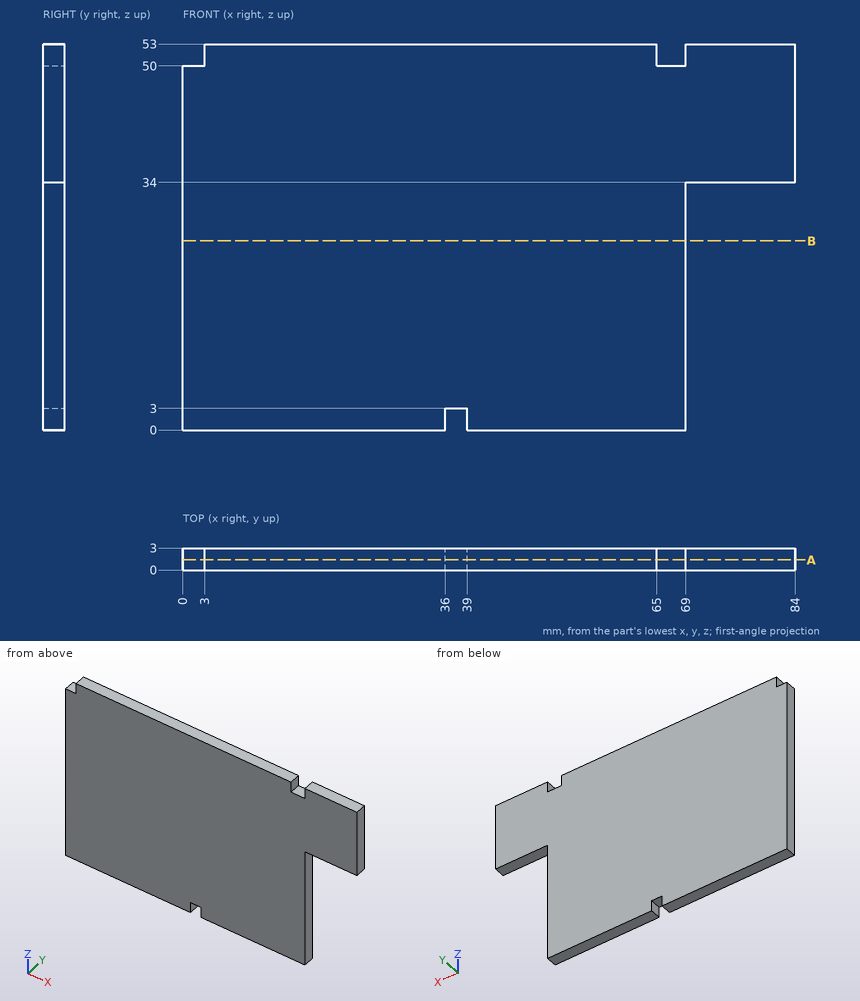
Geometry: see drawing. Coordinates: mm, zero at the bounding-box minimum. Round coordinates to 2 decimals unless told otherwise and drop trailing zeros. Write each loop counter-clockwise with the first axis right and the second up, starting at its lowest first coordinate (ties: lowest second). Pieces come first, ordered by that corner, then holes. Notation, with made-up numbers: M 45,47.25 L 54,47.25 A15 ccw 54,57.25 Z; hole C -27.5,71.25 d5. An arc over 180 degrees is marked long. Answer in a Markdown table with one row per item. Add a question column.
(1) Ray query, L1, parallel to X at y = 2.35, z = 51; L2, parallel to X at y = 2.3, z = 8; L3, parallel to Z at x = 37.5, y = 0.9. Return the intervals inside material, ascending.
(2) Cut plane A-A, the plane y = 1.4. Return the cut outline in (x, z).
(3) Contact query for flat-ended pins moving along their axis: pin 1 (1.5 mm diameter, centred on y = 2, z = 2, fed in from +X); pin 2 (1.5 mm diameter, centred on x = 37.5, y = 1, fed in from -Z); pin 3 (0.9 mm diameter, centred on y = 1, z = 52, fed in from -X); pin 4 (10 mm diameter, centred on x = 46, z = 38, fed in from -Y). Output: stop coordinate, or through.
(4) Cut plane B-B, the plane z = 26. Return the cut outline in (x, y), then the cut area to 3 significant figures.
Established:
| question | item | result |
|---|---|---|
| 1 | L1 | 3 to 65, 69 to 84 |
| 1 | L2 | 0 to 69 |
| 1 | L3 | 3 to 53 |
| 2 | outline | M 0,0 L 36,0 L 36,3 L 39,3 L 39,0 L 69,0 L 69,34 L 84,34 L 84,53 L 69,53 L 69,50 L 65,50 L 65,53 L 3,53 L 3,50 L 0,50 Z |
| 3 | pin 1 | x = 69 |
| 3 | pin 2 | z = 3 |
| 3 | pin 3 | x = 3 |
| 3 | pin 4 | y = 0 |
| 4 | outline | M 0,0 L 69,0 L 69,3 L 0,3 Z |
| 4 | area | 207 mm² |
